Read the model definition and answer for the solid it produces. Units are mm, in the model's axes. A direction names the side the tool comes from. Give positions to 0.01 mm unless a question says otherwise; leave off trailing zeros. Order: outer loops, then holes, each group sorted by start corner. A loop starts at its lowest first (then second) coordinate and runs counter-clockwise, first axis right, second up. Notation, with made-up numbers: (24, 6) - (61, 6) arc R19 cw to (61, 35) - close; hole circle Ø9 at (-34.75, 38). An arc over 180 degrees is marked (long way). Write each question's results on one line, items separated by ' | '. Start each with the question number.
Q1. Find section A-A on z = 0. Give the vertices of the cut face in (x, y).
Q2. A tool of negligible diameter and unlimited length cuts with its end or side. For faces 4 (the face through (-7.81, 8.07, -1.73)), 5 (the face through (-1.2, 1.5, -13.6)), from which of +Z, -Z, +X, -X, +Y, -Y can it reach the whole face along a straight path? Write none if from no direction.
Q3. For a pull along Z with two mould halves and no side action, classify faces 1 (the face through (-15.62, 1.49, -3.47)), 2 (the face through (-10, 2, 0)), 3 (the face through (-5.2, 13, -0.1)) as +Z half, -Z half, draft (parallel to the pull), parting line (faces both ways), or undercut.
Q4. Find the intervals of material crossed by line 1 along Y through (x, z) = (-10.5, -5); line 2 along Z through (x, y) = (0.5, 2.25); line 3 along X through (y, z) = (7.5, 1), in increasing order. Write a range as from..to.
Q5. Find section C-C on y = 9.75. Give the vertices of the cut face in (x, z).
Q6. Flat-ended cylindrical pins translate along their axes: P1, Ø3, axis at y = 10.5, z = -8, coming from the +X side; P2, Ø6, axis at y = 5.5, z = -11, coming from the -X side; P3, Ø2, axis at y = 1.5, z = 4.5, coming from the +X side. Find the tip coordinate at first contact, or state that the pin passes through.
Q7. Find section B-B on x = 0. Give the vertices of the cut face in (y, z).
from build123d import *

# Parameters (mm, degrees)
SKETCH_1_R          = 16
EXTRUDE_1_DEPTH     = 3
SKETCH_2_R          = 2
SKETCH_2_R_2        = 5
CUT_EXTRUDE_1_DEPTH = 3
EXTRUDE_START       = 10
SKETCH_4_R          = 8
SKETCH_4_R_2        = 5
EXTRUDE_2_DEPTH     = 10
FILLET_1_R          = 1


with BuildPart() as part:
    # ｽｹｯﾁ1 → ﾎﾞｽ - 押し出し1 (new body)
    with BuildSketch(Plane(origin=(0, 0, 0), x_dir=(1, 0, 0), z_dir=(0, 1, 0))):
        with Locations(Location((0, 0, 0), (0, 0, 270))):
            Circle(SKETCH_1_R)
    extrude(amount=EXTRUDE_1_DEPTH)

    # ｽｹｯﾁ2 → ｶｯﾄ - 押し出し1 (cut)
    with BuildSketch(Plane(origin=(0, 3, 0), x_dir=(1, 0, 0), z_dir=(0, 1, 0))):
        with Locations(Location((0, 12, 0), (0, 0, 270))):
            Circle(SKETCH_2_R)
        with Locations(Location((12, 0, 0), (0, 0, 270))):
            Circle(SKETCH_2_R)
        with Locations(Location((0, -12, 0), (0, 0, 270))):
            Circle(SKETCH_2_R)
        with Locations(Location((-12, 0, 0), (0, 0, 270))):
            Circle(SKETCH_2_R)
        with Locations(Location((0, 0, 0), (0, 0, 270))):
            Circle(SKETCH_2_R_2)
    extrude(amount=-CUT_EXTRUDE_1_DEPTH, mode=Mode.SUBTRACT)

    # ｽｹｯﾁ4 → ﾎﾞｽ - 押し出し2 (add)
    with BuildSketch(Plane(origin=(0, 3, 0), x_dir=(1, 0, 0), z_dir=(0, 1, 0)).offset(EXTRUDE_START)):
        with Locations(Location((0, 0, 0), (0, 0, 270))):
            Circle(SKETCH_4_R)
        with Locations(Location((0, 0, 0), (0, 0, 270))):
            Circle(SKETCH_4_R_2, mode=Mode.SUBTRACT)
    extrude(amount=-EXTRUDE_2_DEPTH)

    # ﾌｨﾚｯﾄ1
    fillet_1_edges = [part.edges().sort_by_distance(p)[0] for p in [
        (0, 0, -16),
        (0, 3, -16),
    ]]
    fillet(fillet_1_edges, radius=FILLET_1_R)


solid = part.part
Working result:
1) outline: (-16, 1) arc R1 ccw to (-15, 0) - (-14, 0) - (-14, 3) - (-15, 3) arc R1 ccw to (-16, 2) - close; (-10, 0) - (-5, 0) - (-5, 13) - (-8, 13) - (-8, 3) - (-10, 3) - close; (5, 0) - (10, 0) - (10, 3) - (8, 3) - (8, 13) - (5, 13) - close; (14, 0) - (15, 0) arc R1 ccw to (16, 1) - (16, 2) arc R1 ccw to (15, 3) - (14, 3) - close
2) face 4: +Y | face 5: +Y, -Y
3) face 1: parting line | face 2: undercut | face 3: draft
4) line 1: 0..3 | line 2: -15.96..-13.94, -10.06..-4.97, 4.97..10.06, 13.94..15.96 | line 3: -7.94..-4.9, 4.9..7.94
5) outline: circle Ø16 at (0, 0); hole circle Ø10 at (0, 0)
6) P1: x = 4.66 | P2: x = -12.22 | P3: x = 15.61
7) outline: (0, -15) arc R1 ccw to (1, -16) - (2, -16) arc R1 ccw to (3, -15) - (3, -14) - (0, -14) - close; (0, -10) - (3, -10) - (3, -8) - (13, -8) - (13, -5) - (0, -5) - close; (0, 5) - (13, 5) - (13, 8) - (3, 8) - (3, 10) - (0, 10) - close; (0, 14) - (3, 14) - (3, 15) arc R1 ccw to (2, 16) - (1, 16) arc R1 ccw to (0, 15) - close
